Autodesk Inventor part; units mm, degrees
ref_plane "YZ Plane" through (0, 0, 0) normal (1, 0, 0) x (0, 1, 0)
ref_plane "XZ Plane" through (0, 0, 0) normal (0, 1, 0) x (-1, 0, 0)
ref_plane "XY Plane" through (0, 0, 0) normal (0, 0, 1) x (1, 0, 0)
sketch "Sketch1" plane through (0, 0, 0) normal (0, 0, 1) x (1, 0, 0)
  circle A0 centre (0, 0) radius 50
  dimension "d0" = 100
extrude "Extrusion1" add sketch "Sketch1" along normal blind 3
sketch "Sketch2" plane through (0, 0, 3) normal (0, 0, 1) x (1, 0, 0)
  circle A0 centre (0, 0) radius 6.35
  dimension "d3" = 12.7
extrude "Extrusion2" add sketch "Sketch2" along normal blind 30
sketch "Sketch3" plane through (0, 0, 0) normal (0, 0, -1) x (-1, 0, 0)
  circle A0 centre (43.6143, 0) radius 1.5
  circle A1 centre (21.8072, -37.7711) radius 1.5
  circle A2 centre (-21.8072, -37.7711) radius 1.5
  circle A3 centre (-43.6143, 0) radius 1.5
  circle A4 centre (-21.8072, 37.7711) radius 1.5
  circle A5 centre (21.8072, 37.7711) radius 1.5
  point P0 (0, 0)
  dimension "d6" = 3
  dimension "d9" = 360
extrude "Extrusion3" cut sketch "Sketch3" against normal through all
properties part number "Center Lower Disk"
Could you check a few things on this model? Use its own coordinates, in mm. Coordinates: 2 decimals unless noted, no trailing zeros. Loops run counter-clockwise (first coordinate to the right, second up) from the corner with the lowest first, then second, coordinate; pieces in that order, holes last.
1. I need wall thicknesses on L1, parallel to Z at x = 13, y = -2; L2, parallel to X at y = -5.5, z = 6.5; L3, parallel to X at y = -4, z = 19.5. Which ranges of each line are inside material? Lowest first, please.
2. We'd pull the mould along X, two halves only. Please class faces 1 (the face through (-1.38, 6.2, 17.79)), 2 (the face through (0, 0, 33)), 3 (the face through (-21.61, 39.26, 1.48)): released by +X, released by -X, zero draft, split by the parting line, or undercut.
3. Imagine slicing it at D-D (y = 35). Please give me the cut outline in (x, z).
4. Imagine slicing it at A-A (y = 0). Please give me the cut outline in (x, z), and give its area (3 significant figures).
5. For P1, Ø12, axis at y = -26, z = 4.5, coming from the +X side; P2, Ø12, axis at x = -28.5, y = -29, coming from the +Z side; P3, Ø6, axis at x = 23.5, z = 4, coming from the -Y side, each with a flat end and sliding along its axis, tell me the tip position at first contact or that it passes through.
6. Imagine slicing it at B-B (x = 0). Please give me the cut outline in (y, z).
7. Imagine slicing it at C-C (z = 9). Please give me the cut outline in (x, y).
Computed values:
1. L1: z = 0 to 3
1. L2: x = -3.17 to 3.17
1. L3: x = -4.93 to 4.93
2. face 1: split by the parting line
2. face 2: zero draft
2. face 3: undercut
3. outline: (-35.71, 0) - (35.71, 0) - (35.71, 3) - (-35.71, 3) - close
4. outline: (-50, 0) - (-45.11, 0) - (-45.11, 3) - (-50, 3) - close; (-42.11, 0) - (42.11, 0) - (42.11, 3) - (6.35, 3) - (6.35, 33) - (-6.35, 33) - (-6.35, 3) - (-42.11, 3) - close; (45.11, 0) - (50, 0) - (50, 3) - (45.11, 3) - close
4. area: 663 mm2
5. P1: stops at x = 45.74
5. P2: stops at z = 3
5. P3: stops at y = -45.53
6. outline: (-50, 0) - (50, 0) - (50, 3) - (6.35, 3) - (6.35, 33) - (-6.35, 33) - (-6.35, 3) - (-50, 3) - close
7. outline: circle Ø12.7 at (0, 0)
